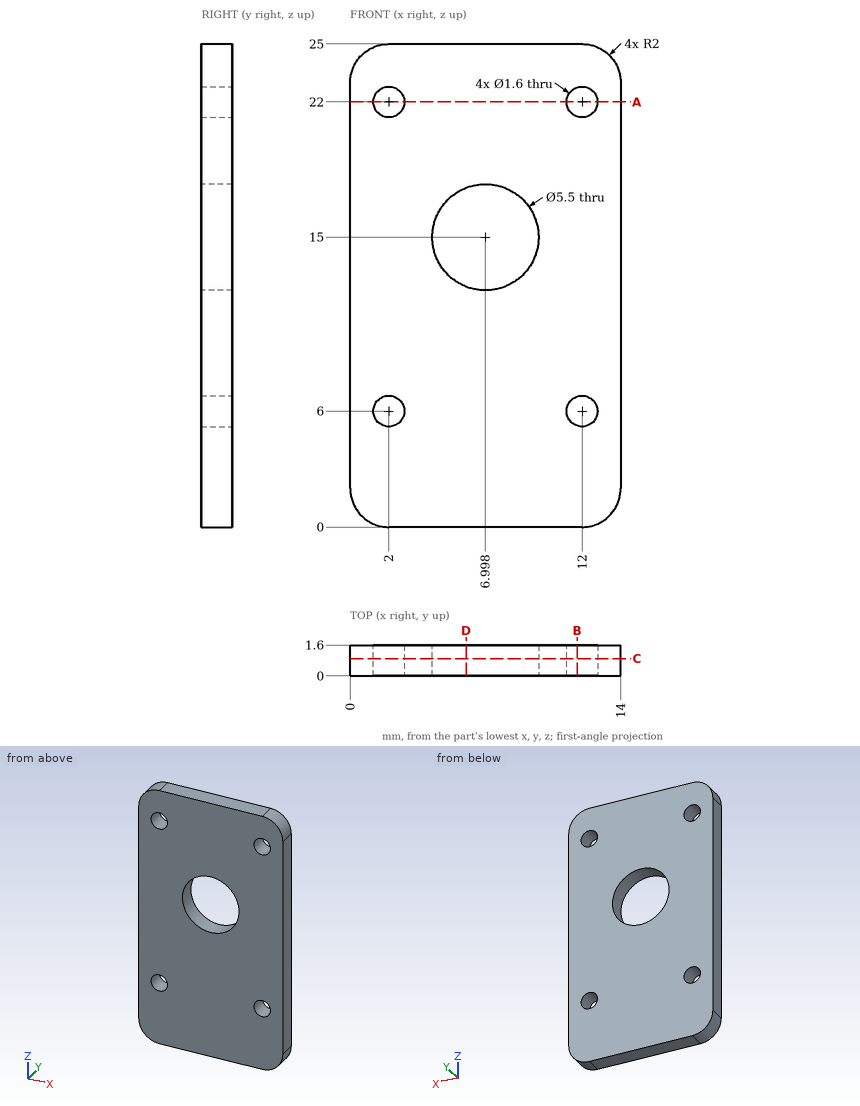
Drawing for the job (mm, zero at the part's lowest x, y, z). Give positions to 0.01 mm unless a question says otherwise; leave off trailing zeros. Write each loop counter-clockwise with the first axis right and the second up, starting at its lowest first coordinate (ties: lowest second). Pieces come first, ordered by that corner, then holes. Notation, with made-up numbers: M 58,14 L 101,14 A5 ccw 101,20 Z; hole C 28,-39.75 d5. An arc over 180 degrees is marked long. Return JSON: item names as keys, results as strings. Group by question number.
(1) Band-saw the part on C-C (y = 0.9). Give the cut face in (x, z), and give its area (3 significant figures).
(2) Flat gauge pin, fed straight in: pin 1 Ø4.5 at (x, z) = (7, 15) entering from -Y. Where does the tip first touch, or does it go through?
(3) Band-saw the part on B-B (x = 11.75). Give the cut face in (y, z).
(4) Band-saw the part on D-D (x = 6). Give the cut face in (y, z).
(5) Band-saw the part on A-A (z = 22). Give the cut face in (x, y).
(6) Drill centre lines: L1, parallel to Z at x = 12, y = 0.55; L2, parallel to X at y = 0.9, z = 22; L3, parallel to Z at x = 6.75, y = 1.05. Where is each one in solid material? Low to high. Write a range as [from, to].
Entries:
{
 "1": {"outline": "M 0,2 A2 ccw 2,0 L 12,0 A2 ccw 14,2 L 14,23 A2 ccw 12,25 L 2,25 A2 ccw 0,23 Z; hole C 2,6 d1.6; hole C 2,22 d1.6; hole C 7,15 d5.5; hole C 12,6 d1.6; hole C 12,22 d1.6", "area": "315 mm^2"},
 "2": {"pin 1": "passes through"},
 "3": {"outline": "M 0,0 L 1.6,0 L 1.6,5.24 L 0,5.24 Z; M 0,6.76 L 1.6,6.76 L 1.6,21.24 L 0,21.24 Z; M 0,22.76 L 1.6,22.76 L 1.6,25 L 0,25 Z"},
 "4": {"outline": "M 0,0 L 1.6,0 L 1.6,12.44 L 0,12.44 Z; M 0,17.56 L 1.6,17.56 L 1.6,25 L 0,25 Z"},
 "5": {"outline": "M 0,0 L 1.2,0 L 1.2,1.6 L 0,1.6 Z; M 2.8,0 L 11.2,0 L 11.2,1.6 L 2.8,1.6 Z; M 12.8,0 L 14,0 L 14,1.6 L 12.8,1.6 Z"},
 "6": {"L1": "z = [0, 5.2], [6.8, 21.2], [22.8, 25]", "L2": "x = [0, 1.2], [2.8, 11.2], [12.8, 14]", "L3": "z = [0, 12.26], [17.74, 25]"}
}
